```python
from build123d import *

# Parameters (mm, degrees)
F0_R          = 15
F3_DEPTH      = 5
F1_R          = 1
F4_DEPTH      = 5
F4_DEPTH_BACK = 1
F2_R          = 2
F5_DEPTH      = 5


with BuildPart() as f3:
    # F0 (on Top) → F3 (new body)
    with BuildSketch(Plane.XY):
        Circle(F0_R)
    extrude(amount=F3_DEPTH)

    # F1 (on Top) → F4 (cut, two sides)
    with BuildSketch(Plane.XY) as f4_sk:
        with Locations((0, 13)):
            Circle(F1_R)
        with Locations((-4.446262, 12.216004)):
            Circle(F1_R)
        with Locations((-8.356239, 9.958578)):
            Circle(F1_R)
        with Locations((-11.25833, 6.5)):
            Circle(F1_R)
        with Locations((-12.802501, 2.257426)):
            Circle(F1_R)
        with Locations((-12.802501, -2.257426)):
            Circle(F1_R)
        with Locations((-11.25833, -6.5)):
            Circle(F1_R)
        with Locations((-8.356239, -9.958578)):
            Circle(F1_R)
        with Locations((-4.446262, -12.216004)):
            Circle(F1_R)
        with Locations((0, -13)):
            Circle(F1_R)
        with Locations((4.446262, -12.216004)):
            Circle(F1_R)
        with Locations((8.356239, -9.958578)):
            Circle(F1_R)
        with Locations((11.25833, -6.5)):
            Circle(F1_R)
        with Locations((12.802501, -2.257426)):
            Circle(F1_R)
        with Locations((12.802501, 2.257426)):
            Circle(F1_R)
        with Locations((11.25833, 6.5)):
            Circle(F1_R)
        with Locations((8.356239, 9.958578)):
            Circle(F1_R)
        with Locations((4.446262, 12.216004)):
            Circle(F1_R)
    extrude(amount=F4_DEPTH, mode=Mode.SUBTRACT)
    extrude(f4_sk.sketch, amount=-F4_DEPTH_BACK, mode=Mode.SUBTRACT)

    # F2 (on Top) → F5 (cut)
    with BuildSketch(Plane.XY):
        Circle(F2_R)
    extrude(amount=F5_DEPTH, mode=Mode.SUBTRACT)


solid = f3.part
```
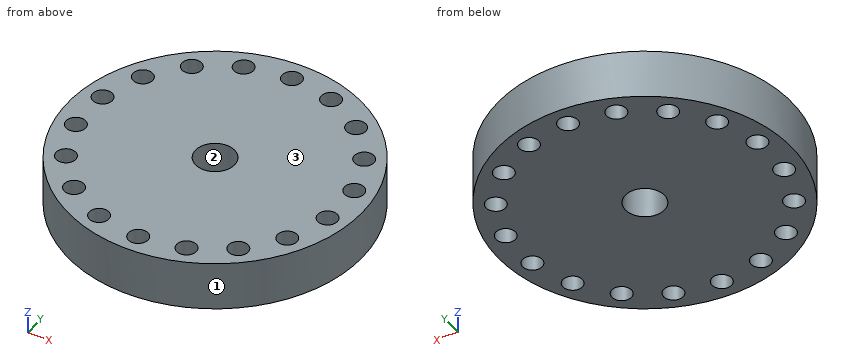
Model file for the job. Use its own axes, mm. Face numbers are marked on the shaded views. Round coordinates to 2 decimals unless told otherwise and drop trailing zeros. Write each loop counter-clockwise with the first axis right and the second up, starting at its lowest first coordinate (ties: lowest second). Pieces come first, ordered by that corner, then holes. Notation, with made-up numbers: (-1, 2) - (43, 2) arc R13 cw to (43, 24) - close; hole circle Ø3 at (-36.75, 22). An arc over 180 degrees is marked (long way). Use CSV: the item, a comma, the result in double quotes. Start each with the question number.
Item 1: Band-saw the part on C-C (y = 0). Write the cut outline in (x, z), and give its area (3 significant figures).
Item 2: Band-saw the part on A-A (x = 0). Write the cut outline in (y, z).
Item 3: Pin check, flat tips, straight feed: P1, Ø3, axis at x = 4.5, z = 3, coming from the -Y side; P2, Ø3, axis at y = -9.5, z = 1.5, coming from the -X side. Stop position of each tip, or through.
Item 4: Band-saw the part on B-B (y = 9.5). Write the cut outline in (x, z).
Item 5: Two-plate mould, pull along Y, no slides. Class the marked faces 1, 2 and 3: released by +Y, released by -Y, zero draft, split by the parting line, or undercut.
Item 6: Drill centre lines: L1, parallel to Y at x = 0, z = 2.55; L2, parallel to Y at x = -4.5, z = 3.15; L3, parallel to Y at x = -12.5, z = 2.2. Where is each one in solid material? Low to high. Write a range as [from, to].
Item 7: Band-saw the part on D-D (x = 8.75). Write the cut outline in (y, z).
Checked values:
1,outline,"(-15, 0) - (-2, 0) - (-2, 5) - (-15, 5) - close; (2, 0) - (15, 0) - (15, 5) - (2, 5) - close"
1,area,"130 mm²"
2,outline,"(-15, 0) - (-14, 0) - (-14, 5) - (-15, 5) - close; (-12, 0) - (-2, 0) - (-2, 5) - (-12, 5) - close; (2, 0) - (12, 0) - (12, 5) - (2, 5) - close; (14, 0) - (15, 0) - (15, 5) - (14, 5) - close"
3,P1,"stops at y = -14.7"
3,P2,"stops at x = -12.69"
4,outline,"(-11.61, 0) - (-9.24, 0) - (-9.24, 5) - (-11.61, 5) - close; (-7.47, 0) - (7.47, 0) - (7.47, 5) - (-7.47, 5) - close; (9.24, 0) - (11.61, 0) - (11.61, 5) - (9.24, 5) - close"
5,face 1,"split by the parting line"
5,face 2,"undercut"
5,face 3,"zero draft"
6,L1,"y = [-15, -14], [-12, -2], [2, 12], [14, 15]"
6,L2,"y = [-14.31, -13.21], [-11.22, 11.22], [13.21, 14.31]"
6,L3,"y = [-8.29, -3.21], [-1.3, 1.3], [3.21, 8.29]"
7,outline,"(-12.18, 0) - (-10.88, 0) - (-10.88, 5) - (-12.18, 5) - close; (-9.04, 0) - (9.04, 0) - (9.04, 5) - (-9.04, 5) - close; (10.88, 0) - (12.18, 0) - (12.18, 5) - (10.88, 5) - close"
